Geometry check sheet. Reference: the model listing, model coordinates, mm. Round coordinates to 2 decimals unless told otherwise and drop trailing zeros. Loops run counter-clockwise (first coordinate to the right, second up) from the corner with the lowest first, then second, coordinate; pieces in that order, holes last. Notation, with made-up numbers: (39.5, 17.5) -> (96.5, 17.5) arc R19 cw to (96.5, 21.5) -> close; hole circle Ø8 at (13, -37.75). An arc over 180 degrees is marked (long way). Use a Markdown table: item, result. Add a question column.
Q1. Sectioned sample at A-A, the plane z = -21.5. Enter the section's corners in (x, y), then the cut area to 4 significant figures.
Q2. Gauge pin test, flat ends, axial feed: P1, Ø0.6, axis at x = 0.5, y = -34, coming from the +Z side; P2, Ø0.8, axis at x = 1, z = 38.5, coming from the -Y side. Record the tip position at first contact, or that the pin passes through.
Q3. Material ranges on L1, parallel to Z at x = 1.25, y = 20.5; L2, parallel to Z at x = 1.3, y = -21; L3, parallel to Y at x = 0.3, z = -14, recorded low to high.
Q4. Sectioned sample at D-D, the plane y = 0. Enter the section's corners in (x, z), then the cut area to 3 significant figures.
Q5. Sectioned sample at C-C, the plane z = 39. Enter the section's corners in (x, y).
Q6. Sectioned sample at B-B, the plane y = 7.5. Enter the section's corners in (x, z).
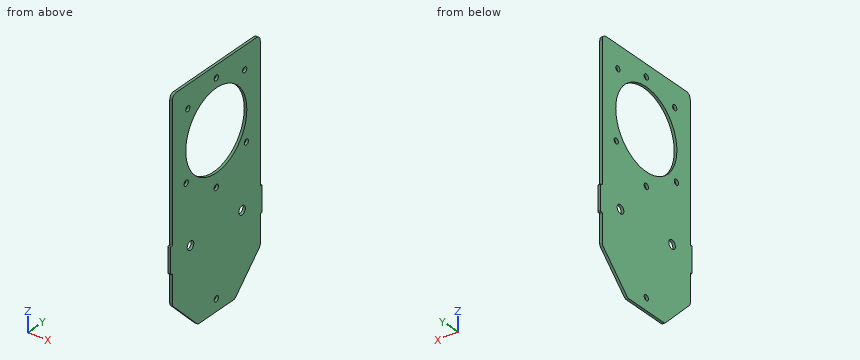
```python
from build123d import *

# Parameters (mm, degrees)
F0_R     = 2.5
F0_R_2   = 1.6
F0_R_3   = 1.65
F0_R_4   = 23.1
F1_DEPTH = 1.5


with BuildPart() as f1:
    # F0 (on Right) → F1 (new body)
    with BuildSketch(Plane.YZ):
        with BuildLine():
            ThreePointArc((33.25, 64), (32.37132, 66.12132), (30.25, 67))
            Line((30.25, 67), (-30.25, 67))
            ThreePointArc((-30.25, 67), (-32.37132, 66.12132), (-33.25, 64))
            Line((-33.25, 64), (-33.25, -14.5))
            ThreePointArc((-33.25, -14.5), (-33.396447, -14.853553), (-33.75, -15))
            Line((-33.75, -15), (-34.25, -15))
            ThreePointArc((-34.25, -15), (-34.603553, -15.146447), (-34.75, -15.5))
            Line((-34.75, -15.5), (-34.75, -29.5))
            ThreePointArc((-34.75, -29.5), (-34.603553, -29.853553), (-34.25, -30))
            Line((-34.25, -30), (-33.75, -30))
            ThreePointArc((-33.75, -30), (-33.396447, -30.146447), (-33.25, -30.5))
            Line((-33.25, -30.5), (-33.25, -46.679121))
            ThreePointArc((-33.25, -46.679121), (-33.100218, -47.438524), (-32.673308, -48.084182))
            Line((-32.673308, -48.084182), (-14.587312, -66.40506))
            ThreePointArc((-14.587312, -66.40506), (-13.935328, -66.845281), (-13.164004, -67))
            Line((-13.164004, -67), (13.164004, -67))
            ThreePointArc((13.164004, -67), (13.935328, -66.845281), (14.587312, -66.40506))
            Line((14.587312, -66.40506), (32.673308, -48.084182))
            ThreePointArc((32.673308, -48.084182), (33.100218, -47.438524), (33.25, -46.679121))
            Line((33.25, -46.679121), (33.25, -30.5))
            ThreePointArc((33.25, -30.5), (33.396447, -30.146447), (33.75, -30))
            Line((33.75, -30), (34.25, -30))
            ThreePointArc((34.25, -30), (34.603553, -29.853553), (34.75, -29.5))
            Line((34.75, -29.5), (34.75, -15.5))
            ThreePointArc((34.75, -15.5), (34.603553, -15.146447), (34.25, -15))
            Line((34.25, -15), (33.75, -15))
            ThreePointArc((33.75, -15), (33.396447, -14.853553), (33.25, -14.5))
            Line((33.25, -14.5), (33.25, 64))
        make_face()
        with Locations((-19.5, -21.5)):
            Circle(F0_R, mode=Mode.SUBTRACT)
        with Locations((0, -60)):
            Circle(F0_R_2, mode=Mode.SUBTRACT)
        with Locations((19.5, -21.5)):
            Circle(F0_R, mode=Mode.SUBTRACT)
        with Locations((-22.75, 14)):
            Circle(F0_R_2, mode=Mode.SUBTRACT)
        with Locations((-21.5, 53.83)):
            Circle(F0_R_2, mode=Mode.SUBTRACT)
        with Locations((0, 0.5)):
            Circle(F0_R_3, mode=Mode.SUBTRACT)
        with Locations((0, 31.5)):
            Circle(F0_R_4, mode=Mode.SUBTRACT)
        with Locations((22.75, 14)):
            Circle(F0_R_2, mode=Mode.SUBTRACT)
        with Locations((0, 60)):
            Circle(F0_R_2, mode=Mode.SUBTRACT)
        with Locations((21.5, 53.83)):
            Circle(F0_R_2, mode=Mode.SUBTRACT)
    extrude(amount=F1_DEPTH)


solid = f1.part
```
Values:
| question | item | result |
|---|---|---|
| 1 | outline | (0, -34.75) -> (1.5, -34.75) -> (1.5, -22) -> (0, -22) -> close; (0, -17) -> (1.5, -17) -> (1.5, 17) -> (0, 17) -> close; (0, 22) -> (1.5, 22) -> (1.5, 34.75) -> (0, 34.75) -> close |
| 1 | area | 89.25 mm^2 |
| 2 | P1 | z = -15 |
| 2 | P2 | y = -33.25 |
| 3 | L1 | -60.42 to -23.79, -19.21 to 20.85, 42.15 to 52.58, 55.08 to 67 |
| 3 | L2 | -59.91 to -23.5, -19.5 to 21.88, 41.12 to 52.31, 55.35 to 67 |
| 3 | L3 | -33.25 to 33.25 |
| 4 | outline | (0, -67) -> (1.5, -67) -> (1.5, -61.6) -> (0, -61.6) -> close; (0, -58.4) -> (1.5, -58.4) -> (1.5, -1.15) -> (0, -1.15) -> close; (0, 2.15) -> (1.5, 2.15) -> (1.5, 8.4) -> (0, 8.4) -> close; (0, 54.6) -> (1.5, 54.6) -> (1.5, 58.4) -> (0, 58.4) -> close; (0, 61.6) -> (1.5, 61.6) -> (1.5, 67) -> (0, 67) -> close |
| 4 | area | 117 mm^2 |
| 5 | outline | (0, -33.25) -> (1.5, -33.25) -> (1.5, -21.85) -> (0, -21.85) -> close; (0, 21.85) -> (1.5, 21.85) -> (1.5, 33.25) -> (0, 33.25) -> close |
| 6 | outline | (0, -67) -> (1.5, -67) -> (1.5, 9.65) -> (0, 9.65) -> close; (0, 53.35) -> (1.5, 53.35) -> (1.5, 67) -> (0, 67) -> close |
